```python
from build123d import *

# Parameters (mm, degrees)
SKETCH4_R           = 5.5
SKETCH6_R           = 3.175
HOLE_SHAFT_DEPTH    = 10
SKETCH7_R           = 3.4
HOLE_POT_DEPTH      = 10
SKETCH8_R           = 2
HOLE_INSERT_DEPTH   = 6.5000001
BOSS_EXTRUDE3_DEPTH = 1.5


with BuildPart() as part:
    # Sweep2: sweep along a path in PROFILE
    with BuildLine(Plane(origin=(0, 0, 0), x_dir=(1, 0, 0), z_dir=(0, 1, 0))) as sweep2_path:
        Line((2.5, -25), (2.5, -10))
        ThreePointArc((2.5, -10), (-0.172829853, -2.126097159), (-7.086656691, 2.49357424))
        Line((-7.086656691, 2.49357424), (-16.745914953, 5.081764691))
    # Sketch4 → Sweep2 (sweep)
    with BuildSketch(Plane.XY.offset(25)):
        with Locations((2.5, 0)):
            Circle(SKETCH4_R)
    sweep(path=sweep2_path.line)

    # Sketch6 → HOLE_SHAFT (cut)
    with BuildSketch(Plane.XY.offset(25)):
        with Locations((2.5, 0)):
            Circle(SKETCH6_R)
    extrude(amount=-HOLE_SHAFT_DEPTH, mode=Mode.SUBTRACT)

    # Sketch7 → HOLE_POT (cut)
    with BuildSketch(Plane(origin=(-16.894592529, 0, -4.526892425), x_dir=(-0.258819045, 0, 0.965925826), z_dir=(-0.965925826, 0, -0.258819045))):
        with Locations((-0.57444604, 0)):
            Circle(SKETCH7_R)
    extrude(amount=-HOLE_POT_DEPTH, mode=Mode.SUBTRACT)

    # Sketch8 → HOLE_INSERT (cut, through all)
    with BuildSketch(Plane(origin=(0, 0, 0), x_dir=(1, 0, 0), z_dir=(0, 1, 0))):
        with Locations((-12.643487424, 3.982522547)):
            Circle(SKETCH8_R)
    extrude(amount=HOLE_INSERT_DEPTH, mode=Mode.SUBTRACT)

    # Sketch11 → Boss-Extrude3 (add)
    with BuildSketch(Plane(origin=(-7.235334266, 0, -1.938701974), x_dir=(-0.258819045, 0, 0.965925826), z_dir=(-0.965925826, 0, -0.258819045))):
        with BuildLine():
            Line((-0.905457853, 3.383848575), (0.72667763, -3.141190411))
            ThreePointArc((0.72667763, -3.141190411), (0.250591719, -3.298380314), (-0.243434227, -3.383848575))
            Line((-0.243434227, -3.383848575), (-1.87556971, 3.141190411))
            ThreePointArc((-1.87556971, 3.141190411), (-1.3994838, 3.298380314), (-0.905457853, 3.383848575))
        make_face()
    extrude(amount=BOSS_EXTRUDE3_DEPTH)


solid = part.part
```
Part model, mm, in its own coordinate system. A direction names the side the tool comes from. Round coordinates to 2 decimals unless told otherwise and drop trailing zeros. Loops run counter-clockwise (first coordinate to the right, second up) from the corner with the lowest first, then second, coordinate; pieces in that order, holes last. Notation, with made-up numbers: (41.25, -12.5) -> (90.25, -12.5) arc R4 ccw to (90.25, -6.5) -> close; hole circle Ø4 at (50.25, 84). An arc over 180 degrees is marked (long way). Use a Markdown table: item, result.
1) Cut at B-B, the plane z = 21. List the corners of the cut face in (x, y) (3 decimals), and give its area (3 significant figures).
The answers:
| item | result |
|---|---|
| outline | circle Ø11 at (2.5, 0); hole circle Ø6.35 at (2.5, 0) |
| area | 63.4 mm2 |
2) Cut at A-A, the plane y = 0. List the corners of the cut face in (x, z) (3 decimals).
The answers:
| item | result |
|---|---|
| outline | (-18.169, 0.231) -> (-17.626, -1.798) -> (-7.967, 0.791) -> (-7.22, -1.996) -> (-8.669, -2.384) -> (-8.402, -3.38) -> (-6.953, -2.991) -> (-6.207, -5.778) -> (-15.866, -8.366) -> (-15.322, -10.394) -> (-5.663, -7.806) arc R18.434 ccw to (8, 10) -> (8, 25) -> (5.675, 25) -> (5.675, 15) -> (-0.675, 15) -> (-0.675, 25) -> (-3, 25) -> (-3, 10) arc R7.434 cw to (-8.51, 2.819) -> close |
3) Drop flat-ended pins along their axis: pin 1 Ø6 at (x, y) = (1.5, 3) entering from -Z; pin 2 Ø5.5 at (x, y) = (2.5, 0) entering from +Z; pin 3 Ø4 at (y, z) = (2, 20) entering from -X; pin 4 Ø6 at (y, z) = (-0.5, 16) entering from +X. Give the stop position or say it passes through.
The answers:
| item | result |
|---|---|
| pin 1 | stops at z = -5.65 |
| pin 2 | stops at z = 15 |
| pin 3 | stops at x = -3 |
| pin 4 | stops at x = 8 |
4) Pull direction X, two halves, no side cores. Call faces 1 (the flat face through (4.9, -2.4, 25)), 2 (the cylindrical face through (-11.22, -4.64, -6.66)), 3 (the cylindrical face through (-0.02, -1.93, 20.07)): pulls with the +X half, pulls with the -X half, needs draft (parallel to the pull), parting line crosses it, or undercut.
The answers:
| item | result |
|---|---|
| face 1 | needs draft |
| face 2 | parting line crosses it |
| face 3 | undercut |
5) Tool access for faces 4 (the flat face through (2, 0, 15)), 5 (the cylindrical face through (-12.904, 4.107, -5.966)), 6 (the flat face through (-7.924, 0.167, -2.227)), 7 (the flat face through (-16.726, 3.59, -5.156)): list every direction of +Z, -Z, +X, -X, +Y, -Y with a clear straight run to the whole face (end or side of a thin tool).
The answers:
| item | result |
|---|---|
| face 4 | +Z |
| face 5 | +Y |
| face 6 | none |
| face 7 | -Z, -X, +Y, -Y |
6) Probe line 1 (Y direction, x = 2.5, z = 18.5) (3 decimals); line 2 (X direction, y = -2, z = 17); line 3 (Y direction, x = 2, z = 7.5). List the from-to ranges inside material, lowest first. Write a range as [from, to].
The answers:
| item | result |
|---|---|
| line 1 | y = [-5.5, -3.175], [3.175, 5.5] |
| line 2 | x = [-2.62, 0.03], [4.97, 7.62] |
| line 3 | y = [-5.49, 5.49] |
